Check sheet for the drawn part. Datum: minimum x, y, z corner. Units: mm. A direction names the side the tool comes from. Round coordinates to 2 decimals unless told otherwise and drop trailing zeros. Order: outer loops, then holes, each group sorted by start corner. A loop starts at its lowest first (then second) coordinate and runs counter-clockwise, first axis right, second up. Notation, with made-up numbers: (58, 34.25) -> (101, 34.25) arc R16 cw to (101, 57.25) -> close; hole circle Ø2 at (24, 11.25). An arc over 180 degrees is marked (long way). Answer in a Markdown table with one row per item.
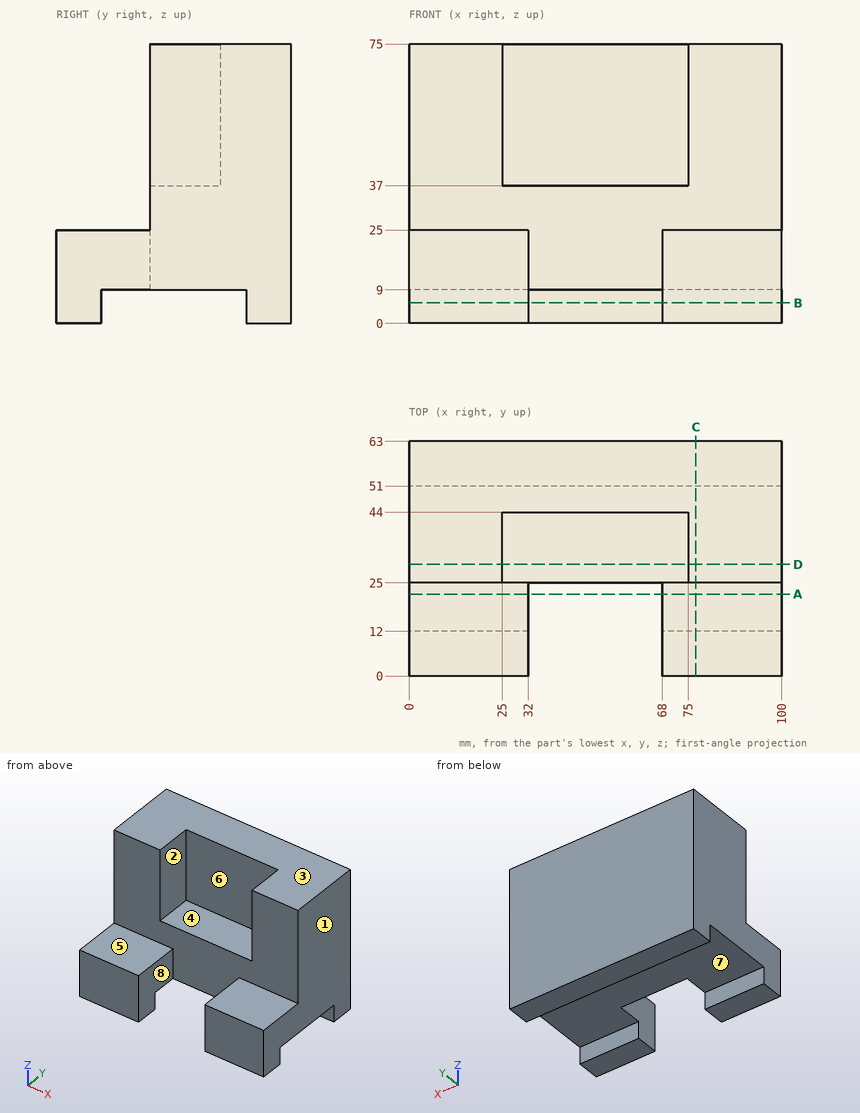
(1) Section check C-C on x = 77. Record the boundary of the cut face in (y, z).
Solutions:
| item | result |
|---|---|
| outline | (0, 0) -> (12, 0) -> (12, 9) -> (51, 9) -> (51, 0) -> (63, 0) -> (63, 75) -> (25, 75) -> (25, 25) -> (0, 25) -> close |
(2) Section check A-A on y = 22. Record the boundary of the cut face in (x, z).
Solutions:
| item | result |
|---|---|
| outline | (0, 9) -> (32, 9) -> (32, 25) -> (0, 25) -> close; (68, 9) -> (100, 9) -> (100, 25) -> (68, 25) -> close |
(3) Tool access check on the marked faces 5, 6, 7 and 8. Record the directions out of +Z, -Z, +X, -X, +Y, -Y that give a thin tool (end or side, any length) a straight path to the whole face; none if there is none.
Solutions:
| item | result |
|---|---|
| face 5 | +Z, +X, -X, -Y |
| face 6 | +Z, -Y |
| face 7 | -Z, +X, -X |
| face 8 | +Z, -Z, -Y |
(4) Draft check along X on the marked faces 1, 2, 3 and 4. Enter one of: pulls with the +X half, pulls with the -X half, needs draft (parallel to the pull), parting line crosses it, or undercut.
Solutions:
| item | result |
|---|---|
| face 1 | pulls with the +X half |
| face 2 | undercut |
| face 3 | needs draft |
| face 4 | undercut |
(5) Section check D-D on y = 30. Record the boundary of the cut face in (x, z), plus the area to 3 significant figures.
Solutions:
| item | result |
|---|---|
| outline | (0, 9) -> (100, 9) -> (100, 75) -> (75, 75) -> (75, 37) -> (25, 37) -> (25, 75) -> (0, 75) -> close |
| area | 4,700 mm^2 |
(6) Scan lines: probe 1 along X at (y, z) = (34, 71); probe 2 along Z at (x, y) = (5, 49); probe 3 along Y at (x, z) = (88.5, 66). Record each from-to range of solid material in increasing order. Write a range as from..to.
Solutions:
| item | result |
|---|---|
| probe 1 | 0..25, 75..100 |
| probe 2 | 9..75 |
| probe 3 | 25..63 |
(7) Depth check by flat-ended pin: pin 1 Ø2 at (x, y) = (85, 36.5) entering from -Z; pin 2 Ø12.5 at (x, y) = (15, 17.5) entering from +Z; pin 3 Ø4 at (x, y) = (60.5, 40) entering from +Z; pin 4 Ø5 at (y, z) = (30, 16) entering from -X. Enter the tip coordinate at first touch or a pass-through.
Solutions:
| item | result |
|---|---|
| pin 1 | z = 9 |
| pin 2 | z = 25 |
| pin 3 | z = 37 |
| pin 4 | x = 0 |
(8) Section check B-B on z = 5.5. Record the boundary of the cut face in (x, y).
Solutions:
| item | result |
|---|---|
| outline | (0, 0) -> (32, 0) -> (32, 12) -> (0, 12) -> close; (0, 51) -> (100, 51) -> (100, 63) -> (0, 63) -> close; (68, 0) -> (100, 0) -> (100, 12) -> (68, 12) -> close |
